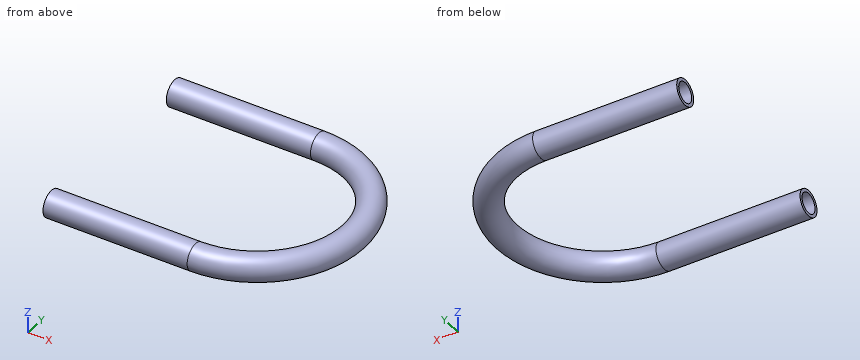
from build123d import *

# Parameters (mm, degrees)
F2_R   = 2.75
F2_R_2 = 2.1


with BuildPart() as f3:
    # F3: sweep along a path in F0
    with BuildLine(Plane.XY) as f3_path:
        Line((-25, 20), (5, 20))
        ThreePointArc((5, 20), (25, 0), (5, -20))
        Line((5, -20), (-25, -20))
    # F2 (on offset) → F3 (sweep)
    with BuildSketch(Plane.YZ.offset(-25)):
        with Locations((20, 0)):
            Circle(F2_R)
        with Locations((20, 0)):
            Circle(F2_R_2, mode=Mode.SUBTRACT)
    sweep(path=f3_path.line)


solid = f3.part
Check sheet for the modelled part. Datum: model origin and axes. Units: mm. Round coordinates to 2 decimals unless told otherwise and drop trailing zeros. Order: outer loops, then holes, each group sorted by start corner. A loop starts at its lowest first (then second) coordinate and runs counter-clockwise, first axis right, second up.
(1) Scan lines: probe 1 along Z at (x, y) = (-2, -20); probe 2 along Y at (x, z) = (13.5, 0.5); probe 3 along Y at (x, z) = (-14.5, 1.4). Record each from-to range of solid material in increasing order.
(2) Cross-section at B-B, the plane x = 1. Enter the section's corners in (y, z), and give its area (3 significant figures).
(3) Go/stop test with flat-tipped pins: P1, Ø8, axis at x = -3.5, y = -11.5, coming from the -Z side; P2, Ø2.5, axis at y = -20, z = 0, coming from the +X side; P3, Ø3, axis at y = -13.5, z = -1.5, coming from the +X side; P4, Ø2, axis at x = -2.5, z = -2, coming from the -Y side. Record where each tip stops, or that it passes through.
(4) Cross-section at A-A, the plane z = 0. Enter the section's corners in (x, y).
Check sheet entries:
1. probe 1: z = -2.75 to -2.1, 2.1 to 2.75
1. probe 2: y = -21.05 to -20.33, -15.82 to -15.06, 15.06 to 15.82, 20.33 to 21.05
1. probe 3: y = -22.37 to -21.57, -18.43 to -17.63, 17.63 to 18.43, 21.57 to 22.37
2. outline: circle Ø5.5 at (-20, 0); circle Ø5.5 at (20, 0); hole circle Ø4.2 at (-20, 0); hole circle Ø4.2 at (20, 0)
2. area: 19.8 mm2
3. P1: passes through
3. P2: stops at x = 17.88
3. P3: stops at x = 24.08
3. P4: stops at y = -22.56
4. outline: (-25, -22.75) - (5, -22.75) arc R22.75 ccw to (5, 22.75) - (-25, 22.75) - (-25, 22.1) - (5, 22.1) arc R22.1 cw to (5, -22.1) - (-25, -22.1) - close; (-25, -17.9) - (5, -17.9) arc R17.9 ccw to (5, 17.9) - (-25, 17.9) - (-25, 17.25) - (5, 17.25) arc R17.25 cw to (5, -17.25) - (-25, -17.25) - close
